```python
from build123d import *

# Parameters (mm, degrees)
SKETCH1_W           = 221
SKETCH1_H           = 6
SKETCH1_W_2         = 5.5
SKETCH1_H_2         = 5.5
BOSS_EXTRUDE1_DEPTH = 232


with BuildPart() as part:
    # Sketch1 → Boss-Extrude1 (new body)
    with BuildSketch(Plane(origin=(0, 0, 0), x_dir=(1, 0, 0), z_dir=(0, 1, 0))):
        with Locations((110.5, 3)):
            Rectangle(SKETCH1_W, SKETCH1_H)
        with Locations((8.75, 3)):
            Rectangle(SKETCH1_W_2, SKETCH1_H_2, mode=Mode.SUBTRACT)
        with Locations((3, 3)):
            Rectangle(SKETCH1_W_2, SKETCH1_H_2, mode=Mode.SUBTRACT)
        with Locations((14.5, 3)):
            Rectangle(SKETCH1_W_2, SKETCH1_H_2, mode=Mode.SUBTRACT)
        with Locations((20.25, 3)):
            Rectangle(SKETCH1_W_2, SKETCH1_H_2, mode=Mode.SUBTRACT)
        with Locations((26, 3)):
            Rectangle(SKETCH1_W_2, SKETCH1_H_2, mode=Mode.SUBTRACT)
        with Locations((31.75, 3)):
            Rectangle(SKETCH1_W_2, SKETCH1_H_2, mode=Mode.SUBTRACT)
        with Locations((37.5, 3)):
            Rectangle(SKETCH1_W_2, SKETCH1_H_2, mode=Mode.SUBTRACT)
        with Locations((43.25, 3)):
            Rectangle(SKETCH1_W_2, SKETCH1_H_2, mode=Mode.SUBTRACT)
        with Locations((49, 3)):
            Rectangle(SKETCH1_W_2, SKETCH1_H_2, mode=Mode.SUBTRACT)
        with Locations((54.75, 3)):
            Rectangle(SKETCH1_W_2, SKETCH1_H_2, mode=Mode.SUBTRACT)
        with Locations((60.5, 3)):
            Rectangle(SKETCH1_W_2, SKETCH1_H_2, mode=Mode.SUBTRACT)
        with Locations((66.25, 3)):
            Rectangle(SKETCH1_W_2, SKETCH1_H_2, mode=Mode.SUBTRACT)
        with Locations((72, 3)):
            Rectangle(SKETCH1_W_2, SKETCH1_H_2, mode=Mode.SUBTRACT)
        with Locations((77.75, 3)):
            Rectangle(SKETCH1_W_2, SKETCH1_H_2, mode=Mode.SUBTRACT)
        with Locations((83.5, 3)):
            Rectangle(SKETCH1_W_2, SKETCH1_H_2, mode=Mode.SUBTRACT)
        with Locations((89.25, 3)):
            Rectangle(SKETCH1_W_2, SKETCH1_H_2, mode=Mode.SUBTRACT)
        with Locations((95, 3)):
            Rectangle(SKETCH1_W_2, SKETCH1_H_2, mode=Mode.SUBTRACT)
        with Locations((100.75, 3)):
            Rectangle(SKETCH1_W_2, SKETCH1_H_2, mode=Mode.SUBTRACT)
        with Locations((106.5, 3)):
            Rectangle(SKETCH1_W_2, SKETCH1_H_2, mode=Mode.SUBTRACT)
        with Locations((112.25, 3)):
            Rectangle(SKETCH1_W_2, SKETCH1_H_2, mode=Mode.SUBTRACT)
        with Locations((118, 3)):
            Rectangle(SKETCH1_W_2, SKETCH1_H_2, mode=Mode.SUBTRACT)
        with Locations((123.75, 3)):
            Rectangle(SKETCH1_W_2, SKETCH1_H_2, mode=Mode.SUBTRACT)
        with Locations((129.5, 3)):
            Rectangle(SKETCH1_W_2, SKETCH1_H_2, mode=Mode.SUBTRACT)
        with Locations((135.25, 3)):
            Rectangle(SKETCH1_W_2, SKETCH1_H_2, mode=Mode.SUBTRACT)
        with Locations((141, 3)):
            Rectangle(SKETCH1_W_2, SKETCH1_H_2, mode=Mode.SUBTRACT)
        with Locations((146.75, 3)):
            Rectangle(SKETCH1_W_2, SKETCH1_H_2, mode=Mode.SUBTRACT)
        with Locations((152.5, 3)):
            Rectangle(SKETCH1_W_2, SKETCH1_H_2, mode=Mode.SUBTRACT)
        with Locations((158.25, 3)):
            Rectangle(SKETCH1_W_2, SKETCH1_H_2, mode=Mode.SUBTRACT)
        with Locations((164, 3)):
            Rectangle(SKETCH1_W_2, SKETCH1_H_2, mode=Mode.SUBTRACT)
        with Locations((169.75, 3)):
            Rectangle(SKETCH1_W_2, SKETCH1_H_2, mode=Mode.SUBTRACT)
        with Locations((175.5, 3)):
            Rectangle(SKETCH1_W_2, SKETCH1_H_2, mode=Mode.SUBTRACT)
        with Locations((181.25, 3)):
            Rectangle(SKETCH1_W_2, SKETCH1_H_2, mode=Mode.SUBTRACT)
        with Locations((187, 3)):
            Rectangle(SKETCH1_W_2, SKETCH1_H_2, mode=Mode.SUBTRACT)
        with Locations((192.75, 3)):
            Rectangle(SKETCH1_W_2, SKETCH1_H_2, mode=Mode.SUBTRACT)
        with Locations((198.5, 3)):
            Rectangle(SKETCH1_W_2, SKETCH1_H_2, mode=Mode.SUBTRACT)
        with Locations((204.25, 3)):
            Rectangle(SKETCH1_W_2, SKETCH1_H_2, mode=Mode.SUBTRACT)
        with Locations((210, 3)):
            Rectangle(SKETCH1_W_2, SKETCH1_H_2, mode=Mode.SUBTRACT)
        with Locations((215.75, 3)):
            Rectangle(SKETCH1_W_2, SKETCH1_H_2, mode=Mode.SUBTRACT)
    extrude(amount=BOSS_EXTRUDE1_DEPTH)


solid = part.part
```
Work out the finished part from the listing and answer in its coordinate system (mm). Give positions to 0.01 mm unless a question says otherwise; leave off trailing zeros. One line per item, written item: value. Start each with the question number.
1. Find section A-A (z = -4.3). State how many separate pieces and enclosed holes the cut face has, and give its area (3 significant figures).
2. Determine the mould class of faces 1 (the face through (132.25, 114, -3)), 2 (the face through (218.5, 114, -3)) for opening direction X: released by +X, released by -X, zero draft, split by the parting line, or undercut.
3. Find the intervals of material crossed by probe 1 along Z at (x, y) = (187.5, 93.5), in increasing order.
4. Each of these flat-tipped pins is pushed along its axis until it touches: P1, Ø3, axis at x = 187.5, z = -1, coming from the +Y side; P2, Ø2, axis at x = 151.5, z = -4, coming from the +Y side. Where does it stop, or does it pass through?
Reported:
1. separate pieces: 39
1. enclosed holes: 0
1. area: 2,780 mm²
2. face 1: undercut
2. face 2: undercut
3. probe 1: z = -6 to -5.75, -0.25 to 0
4. P1: stops at y = 232
4. P2: passes through
